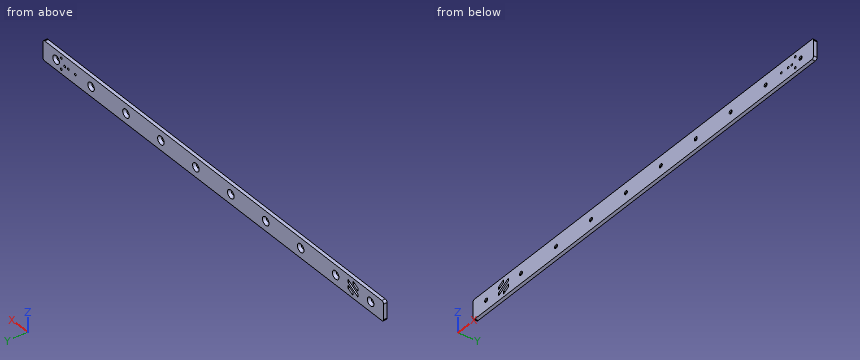
Autodesk Inventor part; units mm, degrees
ref_plane "YZ Plane" through (0, 0, 0) normal (1, 0, 0) x (0, 1, 0)
ref_plane "XZ Plane" through (0, 0, 0) normal (0, 1, 0) x (-1, 0, 0)
ref_plane "XY Plane" through (0, 0, 0) normal (0, 0, 1) x (1, 0, 0)
sketch "ExtrusionBacker_Y_350mm_A" plane through (0, 0, 0) normal (0, 0, 1) x (1, 0, 0)
  circle A0 centre (-11.0001, 28.106) radius 1
  circle A1 centre (-11.0001, 38.106) radius 1
  arc A2 (355.9999, 24.106) -> (357.9999, 26.106) centre (355.9999, 26.106) ccw
  line L0 (357.9999, 26.106) -> (357.9999, 40.106)
  arc A3 (357.9999, 40.106) -> (355.9999, 42.106) centre (355.9999, 40.106) ccw
  line L1 (355.9999, 42.106) -> (-30.0001, 42.106)
  arc A4 (-30.0001, 42.106) -> (-32.0001, 40.106) centre (-30.0001, 40.106) ccw
  line L2 (-32.0001, 40.106) -> (-32.0001, 26.106)
  arc A5 (-32.0001, 26.106) -> (-30.0001, 24.106) centre (-30.0001, 26.106) ccw
  line L3 (-30.0001, 24.106) -> (355.9999, 24.106)
  line L4 (322.9999, 37.0031) -> (328.736, 33.6914)
  line L5 (328.736, 33.6914) -> (328.736, 36.2894)
  line L6 (328.736, 36.2894) -> (322.9999, 39.6012)
  line L7 (322.9999, 39.6012) -> (322.9999, 37.0031)
  line L8 (317.2637, 35.1187) -> (317.2637, 37.7168)
  line L9 (317.2637, 37.7168) -> (328.736, 31.0933)
  line L10 (328.736, 31.0933) -> (328.736, 28.4952)
  line L11 (328.736, 28.4952) -> (317.2637, 35.1187)
  line L12 (317.2637, 32.5207) -> (317.2637, 29.9226)
  line L13 (317.2637, 29.9226) -> (322.9999, 26.6108)
  line L14 (322.9999, 26.6108) -> (322.9999, 29.2089)
  line L15 (322.9999, 29.2089) -> (317.2637, 32.5207)
  circle A6 centre (102.9999, 33.106) radius 1.7
  circle A7 centre (142.9999, 33.106) radius 1.7
  circle A8 centre (222.9999, 33.106) radius 1.7
  circle A9 centre (182.9999, 33.106) radius 1.7
  circle A10 centre (62.9999, 33.106) radius 1.7
  circle A11 centre (302.9999, 33.106) radius 1.7
  circle A12 centre (-3.0001, 33.106) radius 1
  circle A13 centre (342.9999, 33.106) radius 1.7
  circle A14 centre (4.9999, 33.106) radius 1
  circle A15 centre (-17.0001, 33.106) radius 1.7
  circle A16 centre (22.9999, 33.106) radius 1.7
  circle A17 centre (262.9999, 33.106) radius 1.7
  circle A18 centre (-7.0001, 33.106) radius 1
sketch "Skizze1" plane through (0, 0, 0) normal (0, 1, 0) x (-1, 0, 0)
  circle A0 centre (6, -5) radius 1
  circle A1 centre (6, 5) radius 1
  arc A2 (373, -9) -> (375, -7) centre (373, -7) ccw
  line L0 (375, -7) -> (375, 7)
  arc A3 (375, 7) -> (373, 9) centre (373, 7) ccw
  line L1 (373, 9) -> (-13, 9)
  arc A4 (-13, 9) -> (-15, 7) centre (-13, 7) ccw
  line L2 (-15, 7) -> (-15, -7)
  arc A5 (-15, -7) -> (-13, -9) centre (-13, -7) ccw
  line L3 (-13, -9) -> (373, -9)
  line L4 (340, 3.8971) -> (345.7362, 0.5853)
  line L5 (345.7362, 0.5853) -> (345.7362, 3.1834)
  line L6 (345.7362, 3.1834) -> (340, 6.4952)
  line L7 (340, 6.4952) -> (340, 3.8971)
  line L8 (334.2638, 2.0127) -> (334.2638, 4.6108)
  line L9 (334.2638, 4.6108) -> (345.7362, -2.0127)
  line L10 (345.7362, -2.0127) -> (345.7362, -4.6108)
  line L11 (345.7362, -4.6108) -> (334.2638, 2.0127)
  line L12 (334.2638, -0.5853) -> (334.2638, -3.1834)
  line L13 (334.2638, -3.1834) -> (340, -6.4952)
  line L14 (340, -6.4952) -> (340, -3.8971)
  line L15 (340, -3.8971) -> (334.2638, -0.5853)
  circle A6 centre (120, 0) radius 1.7
  circle A7 centre (160, 0) radius 1.7
  circle A8 centre (240, 0) radius 1.7
  circle A9 centre (200, 0) radius 1.7
  circle A10 centre (80, 0) radius 1.7
  circle A11 centre (320, 0) radius 1.7
  circle A12 centre (14, 0) radius 1
  circle A13 centre (360, 0) radius 1.7
  circle A14 centre (22, 0) radius 1
  circle A15 centre (0, 0) radius 1.7
  circle A16 centre (40, 0) radius 1.7
  circle A17 centre (280, 0) radius 1.7
  circle A18 centre (10, 0) radius 1
  point P0 (373, -9)
  point P1 (375, 7)
  point P2 (373, 9)
  point P3 (-13, 9)
  point P4 (-15, 7)
  point P5 (-15, -7)
  point P6 (-13, -9)
  point P7 (334.2638, 2.0127)
  point P8 (334.2638, 4.6108)
  point P9 (345.7362, -2.0127)
  point P10 (345.7362, -4.6108)
  point P11 (340, 3.8971)
  point P12 (340, 6.4952)
  point P13 (345.7362, 0.5853)
  point P14 (340, -3.8971)
  point P15 (340, -6.4952)
  point P16 (334.2638, -3.1834)
  point P17 (334.2638, -0.5853)
extrude "Extrusion1" add sketch "Skizze1" along normal blind 3
sketch "Skizze2" plane through (0, 3, 0) normal (0, 1, 0) x (1, 0, 0)
  circle A0 centre (-360, 0) radius 1.7
  circle A1 centre (-320, 0) radius 1.7
  circle A2 centre (-280, 0) radius 1.7
  circle A3 centre (-240, 0) radius 1.7
  circle A4 centre (-200, 0) radius 1.7
  circle A5 centre (-160, 0) radius 1.7
  circle A6 centre (-120, 0) radius 1.7
  circle A7 centre (-80, 0) radius 1.7
  circle A8 centre (-40, 0) radius 1.7
  circle A9 centre (0, 0) radius 1.7
hole "Bohrung1" at (-360, 3, 0) at (-320, 3, 0) at (-280, 3, 0) at (-240, 3, 0) at (-200, 3, 0) at (-160, 3, 0) at (-120, 3, 0) at (-80, 3, 0) at (-40, 3, 0) at (0, 3, 0) direction (0, -1, 0) diameter 3.4 end through all countersink diameter 7.5 countersink angle 90
properties part number "Y Extrusion-Backer [A] (350mm)" material "Titan"
Geometry check sheet. Reference: the model listing, model coordinates, mm. Coordinates: 2 decimals unless noted, no trailing zeros. Answer in a Markdown table with one row per item. Add a question column.
1) Cross-section at A-A, the plane y = 1.55. State how many separate pieces and enclosed holes the cut face has, then the cut area to 3 significant figures.
2) Material ranges on line 1 along Z through (x, y) = (-6, 0.9); line 2 along X through (y, z) = (0.95, -5.5); line 3 along X through (y, z) = (0.85, 5.25), recorded low to high. Write a range as [from, to].
3) Gauge pin test, flat end, axial feed: P1, Ø4, axis at x = -160, z = 0, coming from the +Y side. Record the tip position at first contact, or that the pin passes through.
Check result:
| question | item | result |
|---|---|---|
| 1 | separate pieces | 1 |
| 1 | enclosed holes | 18 |
| 1 | area | 6,780 mm² |
| 2 | line 1 | z = [-9, -6], [-4, 4], [6, 9] |
| 2 | line 2 | x = [-375, -340], [-338.28, -6.87], [-5.13, 15] |
| 2 | line 3 | x = [-375, -342.16], [-340, -6.97], [-5.03, 15] |
| 3 | P1 | stops at y = 1.25 |
